from build123d import *

# Parameters (mm, degrees)
F0_R     = 19.6
F0_R_2   = 17.6
F0_R_3   = 17
F0_R_4   = 15
F1_DEPTH = 5
F2_DEPTH = 5


with BuildPart() as f1:
    # F0 (on Top) → F1 (new body)
    with BuildSketch(Plane.XY):
        Circle(F0_R)
        Circle(F0_R_2, mode=Mode.SUBTRACT)
        Circle(F0_R_2)
        Circle(F0_R_3, mode=Mode.SUBTRACT)
        Circle(F0_R_3)
        Circle(F0_R_4, mode=Mode.SUBTRACT)
    extrude(amount=-F1_DEPTH)

    # F0 (on Top) → F2 (join)
    with BuildSketch(Plane.XY):
        Circle(F0_R)
        Circle(F0_R_2, mode=Mode.SUBTRACT)
    extrude(amount=F2_DEPTH)


solid = f1.part
Input: part model. Units: mm. Frame: model coordinates. A direction names the side the tool comes from. Round coordinates to 2 decimals unless told otherwise and drop trailing zeros. Write each loop counter-clockwise with the first axis right and the second up, starting at its lowest first coordinate (ties: lowest second). Pieces come first, ordered by that corner, then holes.
1) Ray query, L1, parallel to Y at x = 0, z = -1.8; L2, parallel to Y at x = 0, z = 1.05; L3, parallel to X at y = 0.5, z = 3.75. Return the intervals inside material, ascending.
2) Reachability of faces 3 (the cylindrical face through (16.787, 5.287, 2.465)), 4 (the flat face through (-15, 10, 5)) from +Z, -Z, +X, -X, +Y, -Y: full face, straight path, thin tool, end or side. Return the list, or none.
3) Draft query along Y for faces 1 (the flat face through (13, 8, 0)), 2 (the flat face through (10, -12, -5)). Return one class per face: pulls with the +Y half, pulls with the -Y half, needs draft (parallel to the pull), parting line crosses it, or undercut.
4) Cut plane A-A (x = 0). Return the cut outline in (y, z).
5) Cut plane D-D (y = -15.5). Return the cut outline in (x, z), then the cut area to 3 significant figures.
6) Contact query for flat-ended pins moving along their axis: P1, Ø1, axis at x = 8, z = -1.5, coming from the +Y side; P2, Ø6, axis at y = -7.5, z = 2.5, coming from the -X side; P3, Ø6, axis at y = -8, z = 3.5, coming from the -X side; P4, Ø12, axis at x = -6.5, y = -4, coming from the -Z side. Output: stop coordinate, or through.
7) Cut plane C-C (z = 1.75). Return the cut outline in (x, y).
Geometry says:
1. L1: y = -19.6 to -15, 15 to 19.6
1. L2: y = -19.6 to -17.6, 17.6 to 19.6
1. L3: x = -19.59 to -17.59, 17.59 to 19.59
2. face 3: +Z
2. face 4: +Z, +X, -X, +Y, -Y
3. face 1: undercut
3. face 2: needs draft
4. outline: (-19.6, -5) - (-15, -5) - (-15, 0) - (-17.6, 0) - (-17.6, 5) - (-19.6, 5) - close; (15, -5) - (19.6, -5) - (19.6, 5) - (17.6, 5) - (17.6, 0) - (15, 0) - close
5. outline: (-12, -5) - (12, -5) - (12, 5) - (8.34, 5) - (8.34, 0) - (-8.34, 0) - (-8.34, 5) - (-12, 5) - close
5. area: 157 mm2
6. P1: stops at y = 18.11
6. P2: stops at x = -19.08
6. P3: stops at x = -18.95
6. P4: passes through
7. outline: circle Ø39.2 at (0, 0); hole circle Ø35.2 at (0, 0)
